Check sheet for the modelled part. Datum: model origin and axes. Units: mm. Give positions to 0.01 mm unless a question says otherwise; leave off trailing zeros. Loops run counter-clockwise (first coordinate to the right, second up) from the corner with the lowest first, then second, coordinate; pieces in that order, holes last. Notation, with made-up numbers: (56, 51.5) - (112, 51.5) arc R30 ccw to (112, 82.5) - close; hole circle Ø1 at (-34, -7.5). An arc over 180 degrees is marked (long way). Answer in a Markdown table with one row per item. Add a question column.
(1) Go/stop test with a flat-tipped pin: P1, Ø3, axis at x = 70, y = 0, coming from the -Z side. Record where the tip stops, or that it passes through.
(2) Draft check along Y on faces 1 (the face through (-1, 0, 0)), 2 (the face through (68.331, -0.526, 1.014)). Enter one of: released by +Y, released by -Y, zero draft, split by the parting line, or undercut.
(3) Sectioned sample at A-A on y = 0. Enter the section's corners in (x, z), then the cut area to 3 significant figures.
(4) Thickness scan on L1, parallel to Y at x = 70, z = 0.4; L2, parallel to X at y = -1, z = 0.5; L3, parallel to X at y = 0.5, z = 1.45. Record the ranges inside material, lowest first.
(5) Sectioned sample at B-B on x = -70. Enter the section's corners in (y, z).
from build123d import *

# Parameters (mm, degrees)
SKETCH1_W           = 150
SKETCH1_H           = 20
BOSS_EXTRUDE1_DEPTH = 2
CUT_EXTRUDE1_REACH  = 77.69
SKETCH2_R           = 1.75


with BuildPart() as part:
    # Sketch1 → Boss-Extrude1 (new body)
    with BuildSketch(Plane.XY):
        Rectangle(SKETCH1_W, SKETCH1_H)
    extrude(amount=BOSS_EXTRUDE1_DEPTH)

    # Sketch2 → Cut-Extrude1 (cut, up to next)
    with BuildSketch(Plane.XY.offset(2), mode=Mode.PRIVATE) as cut_extrude1_sk1:
        with Locations((-70, 0)):
            Circle(SKETCH2_R)
    cut_extrude1_tool1 = extrude(cut_extrude1_sk1.sketch, amount=-CUT_EXTRUDE1_REACH, mode=Mode.PRIVATE) & part.part
    # Sketch2 → Cut-Extrude1 (cut, up to next)
    with BuildSketch(Plane.XY.offset(2), mode=Mode.PRIVATE) as cut_extrude1_sk2:
        with Locations(Location((70, 0, 0), (0, 0, 180))):
            Circle(SKETCH2_R)
    cut_extrude1_tool2 = extrude(cut_extrude1_sk2.sketch, amount=-CUT_EXTRUDE1_REACH, mode=Mode.PRIVATE) & part.part
    add(cut_extrude1_tool1.solids().sort_by_distance((-70, 0, 2))[0], mode=Mode.SUBTRACT)
    add(cut_extrude1_tool2.solids().sort_by_distance((70, 0, 2))[0], mode=Mode.SUBTRACT)


solid = part.part
Reply:
| question | item | result |
|---|---|---|
| 1 | P1 | through |
| 2 | face 1 | zero draft |
| 2 | face 2 | undercut |
| 3 | outline | (-75, 0) - (-71.75, 0) - (-71.75, 2) - (-75, 2) - close; (-68.25, 0) - (68.25, 0) - (68.25, 2) - (-68.25, 2) - close; (71.75, 0) - (75, 0) - (75, 2) - (71.75, 2) - close |
| 3 | area | 286 mm^2 |
| 4 | L1 | -10 to -1.75, 1.75 to 10 |
| 4 | L2 | -75 to -71.44, -68.56 to 68.56, 71.44 to 75 |
| 4 | L3 | -75 to -71.68, -68.32 to 68.32, 71.68 to 75 |
| 5 | outline | (-10, 0) - (-1.75, 0) - (-1.75, 2) - (-10, 2) - close; (1.75, 0) - (10, 0) - (10, 2) - (1.75, 2) - close |
